from build123d import *

# Parameters (mm, degrees)
BOSS_EXTRU_1_DEPTH                                = 1.5
BOSS_EXTRU_2_START                                = 0.3
ESQUISSE2_R                                       = 0.83
ESQUISSE2_R_2                                     = 0.87
ESQUISSE2_R_3                                     = 8.2
BOSS_EXTRU_2_DEPTH                                = 3.2
ENL_V_MAT_EXTRU_1_DEPTH                           = 937.37300154
ENL_V_MAT_EXTRU_1_DEPTH_BACK                      = 937.37300154
ESQUISSE1_2_OUTSIDE_W                             = 65.507
ESQUISSE1_2_OUTSIDE_H                             = 36.406
BOSS_EXTRU_3_START                                = 3.2
BOSS_EXTRU_3_DEPTH                                = 3.2
FRAISAGE_POUR_VIS_T_TE_FRAIS_E_BOMB_E_D           = 3.6
FRAISAGE_POUR_VIS_T_TE_FRAIS_E_BOMB_E_CSINK_D     = 6.3
FRAISAGE_POUR_VIS_T_TE_FRAIS_E_BOMB_E_CSINK_ANGLE = 90
ENL_V_MAT_EXTRU_2_DEPTH                           = 118.914346143
ENL_V_MAT_EXTRU_2_DEPTH_BACK                      = 118.914346143
ESQUISSE8_W                                       = 10.000000119
ESQUISSE8_H                                       = 2.5
ESQUISSE9_W                                       = 46.70954475
ESQUISSE9_H                                       = 0.31
ENL_V_MAT_EXTRU_3_DEPTH                           = 10
BOSS_EXTRU_4_DEPTH                                = 3.39
ENL_V_MAT_EXTRU_4_DEPTH                           = 10


with BuildPart() as part:
    # Esquisse1 → Boss.-Extru.1 (new body)
    with BuildSketch(Plane.XZ.offset(51.373319983)):
        with BuildLine():
            Line((-98.670544596, -930.328379496), (-57.379707563, -930.328379496))
            ThreePointArc((-57.379707563, -930.328379496), (-53.577586343, -928.575512729), (-52.441309896, -924.545929189))
            Line((-52.441309896, -924.545929189), (-54.35688847, -912.455846702))
            ThreePointArc((-54.35688847, -912.455846702), (-56.048152904, -909.43617579), (-59.295286137, -908.238297009))
            Line((-59.295286137, -908.238297009), (-96.754966023, -908.238297009))
            ThreePointArc((-96.754966023, -908.238297009), (-100.002099255, -909.43617579), (-101.69336369, -912.455846702))
            Line((-101.69336369, -912.455846702), (-103.608942263, -924.545929189))
            ThreePointArc((-103.608942263, -924.545929189), (-102.472665816, -928.575512729), (-98.670544596, -930.328379496))
        make_face()
    extrude(amount=BOSS_EXTRU_1_DEPTH)

    # Esquisse2 → Boss.-Extru.2 (add)
    with BuildSketch(Plane.XY.offset(-911.638297009).offset(BOSS_EXTRU_2_START)):
        with BuildLine():
            Line((-52.906931145, -51.073319983), (-52.906931145, -31.173319983))
            ThreePointArc((-52.906931145, -31.173319983), (-53.77096614, -29.087354978), (-55.856931145, -28.223319983))
            Line((-55.856931145, -28.223319983), (-100.656931145, -28.223319983))
            ThreePointArc((-100.656931145, -28.223319983), (-102.742896149, -29.087354978), (-103.606931145, -31.173319983))
            Line((-103.606931145, -31.173319983), (-103.606931145, -51.073319983))
            Line((-103.606931145, -51.073319983), (-103.608942263, -51.373319983))
            Line((-103.608942263, -51.373319983), (-52.906931145, -51.373319983))
            Line((-52.906931145, -51.373319983), (-52.906931145, -51.073319983))
        make_face()
        with Locations((-99.356931145, -32.373319983)):
            Circle(ESQUISSE2_R, mode=Mode.SUBTRACT)
        with Locations((-99.356931145, -49.873319983)):
            Circle(ESQUISSE2_R_2, mode=Mode.SUBTRACT)
        with Locations((-57.156931145, -49.873319983)):
            Circle(ESQUISSE2_R_2, mode=Mode.SUBTRACT)
        with Locations((-57.156931145, -32.373319983)):
            Circle(ESQUISSE2_R_2, mode=Mode.SUBTRACT)
        with Locations((-91.256931145, -41.073319983)):
            Circle(ESQUISSE2_R_3, mode=Mode.SUBTRACT)
        with Locations((-65.256931145, -41.073319983)):
            Circle(ESQUISSE2_R_3, mode=Mode.SUBTRACT)
    extrude(amount=BOSS_EXTRU_2_DEPTH)

    # Esquisse1_2 outside → Enl_v. mat.-Extru.1 (cut, two sides: drawn at the far end of the back side and taken through both)
    with BuildSketch(Plane.XZ.offset(51.373319983).offset(-ENL_V_MAT_EXTRU_1_DEPTH_BACK)):
        with Locations((-78.0255, -919.233)):
            Rectangle(ESQUISSE1_2_OUTSIDE_W, ESQUISSE1_2_OUTSIDE_H)
        with BuildLine():
            Line((-98.670544596, -930.328379496), (-57.379707563, -930.328379496))
            ThreePointArc((-57.379707563, -930.328379496), (-53.577586343, -928.575512729), (-52.441309896, -924.545929189))
            Line((-52.441309896, -924.545929189), (-54.35688847, -912.455846702))
            ThreePointArc((-54.35688847, -912.455846702), (-56.048152904, -909.43617579), (-59.295286137, -908.238297009))
            Line((-59.295286137, -908.238297009), (-96.754966023, -908.238297009))
            ThreePointArc((-96.754966023, -908.238297009), (-100.002099255, -909.43617579), (-101.69336369, -912.455846702))
            Line((-101.69336369, -912.455846702), (-103.608942263, -924.545929189))
            ThreePointArc((-103.608942263, -924.545929189), (-102.472665816, -928.575512729), (-98.670544596, -930.328379496))
        make_face(mode=Mode.SUBTRACT)
    extrude(amount=ENL_V_MAT_EXTRU_1_DEPTH + ENL_V_MAT_EXTRU_1_DEPTH_BACK, mode=Mode.SUBTRACT)

    # Esquisse3 → Boss.-Extru.3 (add)
    with BuildSketch(Plane(origin=(0, -51.373319983, 0), x_dir=(1, 0, 0), z_dir=(0, 1, 0)).offset(BOSS_EXTRU_3_START)):
        with BuildLine():
            ThreePointArc((-102.982508149, 927.859578881), (-103.376352569, 927.018163899), (-103.607735067, 926.118411302))
            ThreePointArc((-103.607735067, 926.118411302), (-94.922727103, 921.708622836), (-85.517242835, 919.176338626))
            ThreePointArc((-85.517242835, 919.176338626), (-84.485661398, 919.92188523), (-85.231208003, 920.953466667))
            ThreePointArc((-85.231208003, 920.953466667), (-94.473289986, 923.464655248), (-102.982508149, 927.859578881))
        make_face()
        with BuildLine():
            ThreePointArc((-71.253122945, 919.966173311), (-61.614344657, 922.608295593), (-52.765422079, 927.254092215))
            ThreePointArc((-52.765422079, 927.254092215), (-53.176239028, 928.035934163), (-53.718212164, 928.733295272))
            ThreePointArc((-53.718212164, 928.733295272), (-53.866494414, 928.670740496), (-54.005911098, 928.59034327))
            ThreePointArc((-54.005911098, 928.59034327), (-62.407028515, 924.230869883), (-71.539157777, 921.743301352))
            ThreePointArc((-71.539157777, 921.743301352), (-72.284704381, 920.711719915), (-71.253122945, 919.966173311))
        make_face()
    extrude(amount=-BOSS_EXTRU_3_DEPTH)

    # Fraisage pour vis _ t_te frais_e bomb_e (through all)
    with Locations(Plane.XZ.offset(52.873319983)):
        with Locations((-78.416666646, -918.775310047)):
            CounterSinkHole(FRAISAGE_POUR_VIS_T_TE_FRAIS_E_BOMB_E_D / 2, FRAISAGE_POUR_VIS_T_TE_FRAIS_E_BOMB_E_CSINK_D / 2, counter_sink_angle=FRAISAGE_POUR_VIS_T_TE_FRAIS_E_BOMB_E_CSINK_ANGLE)

    # Esquisse8 → Enl_v. mat.-Extru.2 (cut, two sides: drawn at the far end of the back side and taken through both)
    with BuildSketch(Plane(origin=(0, 0, -911.338297009), x_dir=(-1, 0, 0), z_dir=(0, 0, -1)).offset(-ENL_V_MAT_EXTRU_2_DEPTH_BACK)):
        with Locations((78.256931086, -32.623319983)):
            Rectangle(ESQUISSE8_W, ESQUISSE8_H)
    extrude(amount=ENL_V_MAT_EXTRU_2_DEPTH + ENL_V_MAT_EXTRU_2_DEPTH_BACK, mode=Mode.SUBTRACT)

    # Esquisse9 → Enl_v. mat.-Extru.3 (cut)
    with BuildSketch(Plane.XY.offset(-908.238297009)):
        with Locations((-78.02512608, -51.218319983)):
            Rectangle(ESQUISSE9_W, ESQUISSE9_H)
    extrude(amount=-ENL_V_MAT_EXTRU_3_DEPTH, mode=Mode.SUBTRACT)


with BuildPart() as enl_v_mat_extru_3_piece_1:
    # of the separate pieces the step leaves, piece 1, a body of its own (enl_v_mat_extru_3_pieces)
    add(part.part.solids().sort_by_distance((-101.69336369, -51.373319983, -912.455846702))[0])



with BuildPart() as enl_v_mat_extru_3_piece_2:
    # of the separate pieces the step leaves, piece 2, a body of its own (enl_v_mat_extru_3_pieces)
    add(part.part.solids().sort_by_distance((-96.754966023, -51.063319983, -908.238297009))[0])


with BuildPart() as enl_v_mat_extru_3_piece_2_1:
    # Corps-D_placer_Copier1: moved
    add(enl_v_mat_extru_3_piece_2.part.moved(Location((0, 2.89, 0))))


with BuildPart() as enl_v_mat_extru_3_piece_1_1:
    add(enl_v_mat_extru_3_piece_1.part)

    add(enl_v_mat_extru_3_piece_2_1.part)  # Boss.-Extru.4 merges Enl_v. mat.-Extru.3 piece 2
    # Esquisse10 → Boss.-Extru.4 (add)
    with BuildSketch(Plane.XZ.offset(48.173319983)):
        with BuildLine():
            Line((-59.295286137, -908.238297009), (-96.754966023, -908.238297009))
            ThreePointArc((-96.754966023, -908.238297009), (-99.538848204, -909.084985078), (-101.379898455, -911.338297009))
            Line((-101.379898455, -911.338297009), (-54.670353705, -911.338297009))
            ThreePointArc((-54.670353705, -911.338297009), (-56.511403955, -909.084985078), (-59.295286137, -908.238297009))
        make_face()
    extrude(amount=BOSS_EXTRU_4_DEPTH)

    # Esquisse11 → Enl_v. mat.-Extru.4 (cut)
    with BuildSketch(Plane.XY.offset(-908.238297009)):
        with BuildLine():
            Line((-81.456931145, -43.283319983), (-75.056931145, -43.283319983))
            ThreePointArc((-75.056931145, -43.283319983), (-73.006931145, -45.333319983), (-75.056931145, -47.383319983))
            Line((-75.056931145, -47.383319983), (-81.456931145, -47.383319983))
            ThreePointArc((-81.456931145, -47.383319983), (-83.506931145, -45.333319983), (-81.456931145, -43.283319983))
        make_face()
    extrude(amount=-ENL_V_MAT_EXTRU_4_DEPTH, mode=Mode.SUBTRACT)


solid = enl_v_mat_extru_3_piece_1_1.part
Could you check a few things on this model? Use its own coordinates, in mm. A direction names the side the tool comes from. Round coordinates to 2 decimals unless told otherwise and drop trailing zeros. Order: outer loops, then holes, each group sorted by start corner. A loop starts at its lowest first (then second) coordinate and runs counter-clockwise, first axis right, second up. Notation, with made-up numbers: M -37,58.5 L 9,58.5 A19 cw 9,94.5 Z; hole C 85.5,70.5 d3. An arc over 180 degrees is marked long. One line per item, written item: value.
(1) Imagine slicing it at A-A (y = -41.75). Write out the boundary of the cut face in (x, z).
Ans:
outline: M -101.38,-911.34 L -98.64,-911.34 L -98.64,-908.61 A5 ccw Z; M -83.87,-911.34 L -72.64,-911.34 L -72.64,-908.24 L -83.87,-908.24 Z; M -57.87,-911.34 L -54.67,-911.34 A5 ccw -57.87,-908.44 Z
(2) If we mould it in two halves opening along X, with no side actions, what happens to faces 4 (the flat face through (-78, -52, -930.328)), 5 (the flat face through (-53.386, -52.113, -918.586)), 6 (the cylindrical face through (-73.45, -37.82, -909.81)), 7 (the cylindrical face through (-83.506, -45.378, -909.767))? For each: released by +X, released by -X, zero draft, split by the parting line, or undercut.
Ans:
face 4: zero draft
face 5: released by +X
face 6: undercut
face 7: undercut
(3) I'm going to push flat-ended pins straight in: P1, Ø2, axis at y = -29.5, z = -910.5, coming from the +X side; P2, Ø1, axis at y = -49.5, z = -912, coming from the -X side; P3, Ø9.5, axis at x = -92, z = -922, coming from the +Y side; P4, Ø3, axis at x = -57.16, y = -29.48, coming from the +Z side. Where does each tip first touch, or does it pass through?
Ans:
P1: stops at x = -54.67
P2: passes through
P3: stops at y = -48.17
P4: stops at z = -908.28
(4) I need wall thicknesses on line 1 along Y through (x, z) = (-82.5, -911); line 2 along Y through (x, z) = (-65, -910); line 3 along X through (y, z) = (-47, -910.5). Which ranges of each line are inside material? Lowest first, please. Write a range as from..to.
Ans:
line 1: y = -52.87..-47.1, -43.57..-30.98, -28.48..-25.33
line 2: y = -52.87..-46.38, -29.99..-25.33
line 3: x = -100.94..-100.23, -98.49..-82.65, -73.86..-58.03, -56.29..-55.11
(5) Which directions (+Z, -Z, +X, -X, +Y, -Y) give clear straight access to the entire face, cutting with the end or side of a thin tool? Please do faces 1 (the cylindrical face through (-72.288, -49.751, -920.731)), 2 (the flat face through (-78, -43.283, -910)), 3 (the flat face through (-78, -38, -911.338)).
Ans:
face 1: +Y
face 2: +Z, -Z
face 3: +X, -X, +Y
(6) Imagine slicing it at B-B (x = -92.5). Write out the boundary of the cut face in (y, z).
Ans:
outline: M -52.87,-930.33 L -51.37,-930.33 L -51.37,-922.75 L -48.17,-922.75 L -48.17,-920.85 L -51.37,-920.85 L -51.37,-911.34 L -46.29,-911.34 L -46.29,-908.24 L -52.87,-908.24 Z; M -30.08,-911.34 L -25.33,-911.34 L -25.33,-908.24 L -30.08,-908.24 Z
(7) Imagine slicing it at D-D (z = -925.25). Write out the boundary of the cut face in (x, y), and give its area (3 significant figures).
Ans:
outline: M -103.67,-52.87 L -52.38,-52.87 L -52.38,-51.37 L -56.03,-51.37 L -56.03,-48.17 L -60.01,-48.17 L -60.01,-51.37 L -98.48,-51.37 L -98.48,-48.17 L -102.21,-48.17 L -102.21,-51.37 L -103.67,-51.37 Z
area: 102 mm^2
(8) Imagine slicing it at C-C (y = -45.25). Write out the boundary of the cut face in (x, z).
Ans:
outline: M -101.38,-911.34 L -95.42,-911.34 L -95.42,-908.24 L -96.75,-908.24 A5 ccw Z; M -87.1,-911.34 L -83.51,-911.34 L -83.51,-908.24 L -87.1,-908.24 Z; M -73.01,-911.34 L -69.42,-911.34 L -69.42,-908.24 L -73.01,-908.24 Z; M -61.1,-911.34 L -54.67,-911.34 A5 ccw -59.3,-908.24 L -61.1,-908.24 Z
